from build123d import *

# Parameters (mm, degrees)
SKETCH002_R   = 1.5
SKETCH002_R_2 = 1
PAD002_DEPTH  = 3
SKETCH001_R   = 1
SKETCH001_R_2 = 1.5
PAD001_DEPTH  = 5


with BuildPart() as platte3:
    # Sketch002 → Pad002 (new body)
    with BuildSketch(Plane.XY):
        Polygon((-31.35, 69.37), (-31.35, 0), (-10, 0), (-10, 5), (10, 5), (10, 0), (31.35, 0), (31.35, 69.37), align=None)
        with Locations((-25.17, 62.47)):
            Circle(SKETCH002_R, mode=Mode.SUBTRACT)
        with Locations((25.17, 62.47)):
            Circle(SKETCH002_R, mode=Mode.SUBTRACT)
        with Locations((-28.5, 36.37)):
            Circle(SKETCH002_R, mode=Mode.SUBTRACT)
        with Locations((28.5, 36.37)):
            Circle(SKETCH002_R, mode=Mode.SUBTRACT)
        with Locations((-15, 2.5)):
            Circle(SKETCH002_R, mode=Mode.SUBTRACT)
        with Locations((15, 2.5)):
            Circle(SKETCH002_R, mode=Mode.SUBTRACT)
        with Locations((0, 36.37)):
            Circle(SKETCH002_R_2, mode=Mode.SUBTRACT)
        Polygon((-19, 55.56), (-19, 17.96), (-3, 17.96), (-3, 39.36), (3, 39.36), (3, 17.96), (19, 17.96), (19, 55.56), align=None, mode=Mode.SUBTRACT)
    extrude(amount=PAD002_DEPTH)


with BuildPart() as base_fusion:
    # Sketch001 → Pad001 (new body)
    with BuildSketch(Plane.XY):
        Polygon((-31.35, 69.37), (-31.35, 39.9), (-21.05, 39.9), (-21.05, 0), (-9.89, 0), (-9.89, 5), (9.89, 5), (9.89, 0), (21.05, 0), (21.05, 39.9), (31.35, 39.9), (31.35, 69.37), align=None)
        with Locations((0, 36.37)):
            Circle(SKETCH001_R, mode=Mode.SUBTRACT)
        with Locations((-14.89, 2.5)):
            Circle(SKETCH001_R_2, mode=Mode.SUBTRACT)
        with Locations((14.89, 2.5)):
            Circle(SKETCH001_R_2, mode=Mode.SUBTRACT)
        with Locations((-25.17, 62.46)):
            Circle(SKETCH001_R_2, mode=Mode.SUBTRACT)
        with Locations((25.17, 62.46)):
            Circle(SKETCH001_R_2, mode=Mode.SUBTRACT)
        Polygon((-19, 55.56), (-19, 17.96), (-3, 17.96), (-3, 39.37), (3, 39.37), (3, 17.96), (19, 17.96), (19, 55.56), align=None, mode=Mode.SUBTRACT)
    extrude(amount=PAD001_DEPTH)


with BuildPart() as base_fusion_1:
    # Body001 placement: moved
    add(base_fusion.part.moved(Location((0, 0, 3))))

    # Fusion: union platte3
    add(platte3.part)


with BuildPart() as base_fusion_2:
    # Clone placement: moved
    add(base_fusion_1.part.moved(Location((31.35, 0, -8))))


solid = base_fusion_2.part
Here's how the part is built. I have some questions about the finished solid (model axes, mm). A direction names the side the tool comes from. Coordinates: 2 decimals unless noted, no trailing zeros. Order: outer loops, then holes, each group sorted by start corner. A loop starts at its lowest first (then second) coordinate and runs counter-clockwise, first axis right, second up.
Item 1: If we section it at C-C on y = 21.5: List the corners of the cut face in (x, z) for me, plus the area to 3 significant figures.
Result sheet:
outline: (0, -8) - (12.35, -8) - (12.35, 0) - (10.3, 0) - (10.3, -5) - (0, -5) - close; (28.35, -8) - (34.35, -8) - (34.35, 0) - (28.35, 0) - close; (50.35, -8) - (62.7, -8) - (62.7, -5) - (52.4, -5) - (52.4, 0) - (50.35, 0) - close
area: 143 mm2
Item 2: If we section it at D-D on x = 59.85: List the corners of the cut face in (y, z) for me.
Result sheet:
outline: (0, -8) - (34.87, -8) - (34.87, -5) - (0, -5) - close; (37.87, -8) - (69.37, -8) - (69.37, 0) - (39.9, 0) - (39.9, -5) - (37.87, -5) - close
Item 3: I need wall thicknesses on line 1 (X direction, y = 62.47, z = -5.95); line 2 (Y direction, x = 31.35, z = -3); line 3 (Y direction, x = 46.35, z = -7.1). Which ranges of each line are inside material? Lowest first, please.
Result sheet:
line 1: x = 0 to 4.68, 7.68 to 55.02, 58.02 to 62.7
line 2: y = 5 to 35.37, 37.37 to 39.37, 55.56 to 69.37
line 3: y = 0 to 1, 4 to 17.96, 55.56 to 69.37
Item 4: For P1, Ø0.8, axis at x = 5.5, y = 62, coming from the +Z side; P2, Ø4, axis at x = 31.5, z = -3.5, coming from the -Y side; P3, Ø2, axis at x = 56.5, y = 11, coming from the +Z side; P4, Ø3, axis at x = 56, z = -3, coming from the -Y side, each with a flat end and sliding along its axis, tell me the tip position at first contact or that it passes through.
Result sheet:
P1: passes through
P2: stops at y = 5
P3: stops at z = -5
P4: stops at y = 39.9
Item 5: If we section it at B-B on z = -4: List the corners of the cut face in (x, y) for me, plus the area to 3 significant figures.
Result sheet:
outline: (0, 39.9) - (10.3, 39.9) - (10.3, 0) - (21.46, 0) - (21.46, 5) - (41.24, 5) - (41.24, 0) - (52.4, 0) - (52.4, 39.9) - (62.7, 39.9) - (62.7, 69.37) - (0, 69.37) - close; hole circle Ø3 at (6.18, 62.46); hole (12.35, 17.96) - (28.35, 17.96) - (28.35, 39.37) - (34.35, 39.37) - (34.35, 17.96) - (50.35, 17.96) - (50.35, 55.56) - (12.35, 55.56) - close; hole circle Ø3 at (16.46, 2.5); hole circle Ø2 at (31.35, 36.37); hole circle Ø3 at (46.24, 2.5); hole circle Ø3 at (56.52, 62.46)
area: 2,100 mm2
Item 6: For faces 1 (the face through (20, 17.96, -4)), 2 (the face through (10.3, 20, -3)), 3 (the face through (41.24, 3, -3)), 4 (the face through (57, 20, -5)), 5 (the face through (47.67, 2.95, -2.54)), which set-ups out of +Z, -Z, +X, -X, +Y, -Y let a thin tool reach every point of the face, with its end or its side?
Result sheet:
face 1: +Z, -Z
face 2: +Z, -X, -Y
face 3: +Z, -Z, -Y
face 4: +Z, +X, -Y
face 5: +Z
Item 7: If we mould it in two halves opening along X, with no side actions, what happens to faces 6 (the face through (5, 20, -5)), 7 (the face through (52.4, 20, -3)), 8 (the face through (31, 39.36, -7))? For each: +X half, -X half, draft (parallel to the pull), parting line (faces both ways), or undercut.
Result sheet:
face 6: draft
face 7: +X half
face 8: undercut
